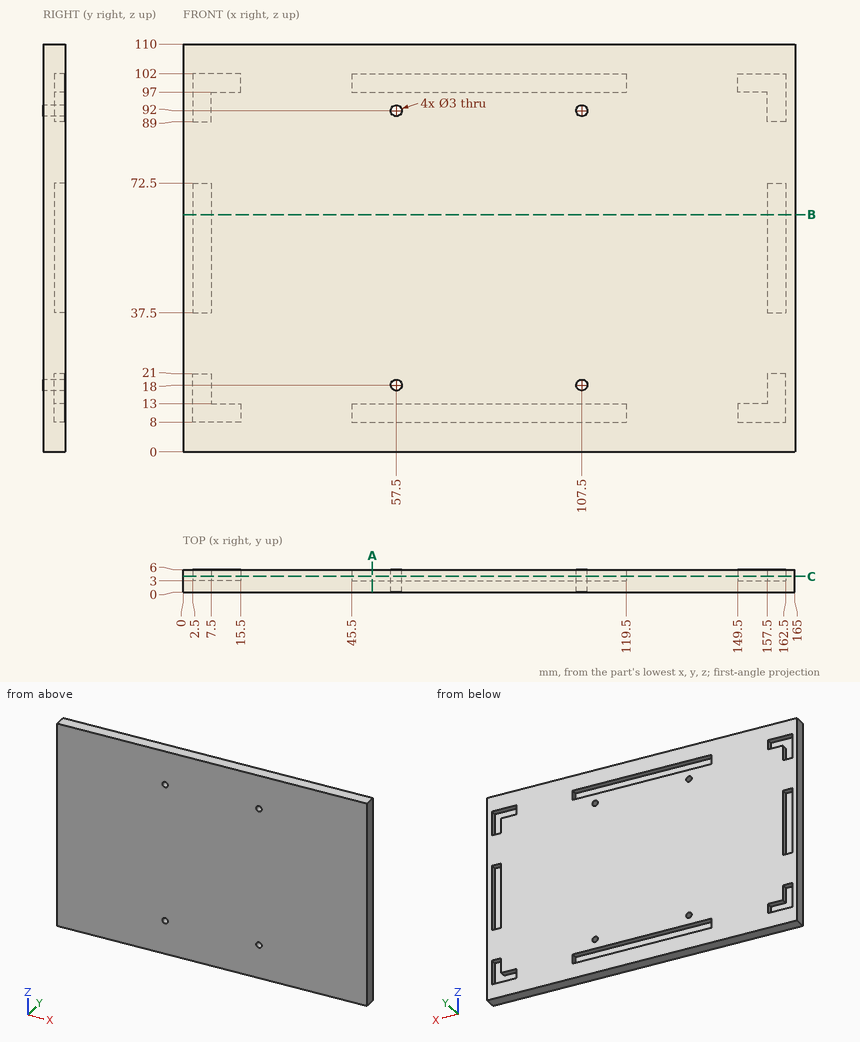
Print and shaded views of the part. All mm, measured from the part's lowest x, y and z. Coordinates: 2 decimals unless noted, no trailing zeros. Loops run counter-clockwise (first coordinate to the right, second up) from the corner with the lowest first, then second, coordinate; pieces in that order, holes last. Notation, with made-up numbers: (40, 75.5) -> (72, 75.5) arc R18 cw to (72, 81.5) -> close; hole circle Ø8 at (50, 37). An arc over 180 degrees is marked (long way). Use one line per item in the form item = value. Start each with the question number.
(1) Flat gauge pin, fed straight in: pin 1 (2.5 mm diameter, centred on x = 76, z = 11, fed in from +Y). Where does the tip first touch, or does it go through?
(2) Probe probe 1 along X at (y, z) = (3.45, 18); probe 2 along X at (y, z) = (2.95, 18); probe 3 along Z at (x, y) = (107.5, 2.4). List the from-to ranges inside material, lowest first. Write a range as from..to.
(3) Cut at B-B on z = 64. Give the cut face in (x, y), and give its area (3 significant figures).
(4) Cut at A-A on x = 51. Give the cut face in (y, z).
(5) Cut at C-C on y = 4.25. Give the number of separate pieces and of enclosed holes in the cut face, and give its area (3 significant figures).
Values:
q1.pin_1 = 3
q2.probe_1 = 0..2.5, 7.5..56, 59..106, 109..157.5, 162.5..165
q2.probe_2 = 0..56, 59..106, 109..165
q2.probe_3 = 0..16.5, 19.5..90.5, 93.5..110
q3.outline = (0, 0) -> (165, 0) -> (165, 6) -> (162.5, 6) -> (162.5, 3) -> (157.5, 3) -> (157.5, 6) -> (7.5, 6) -> (7.5, 3) -> (2.5, 3) -> (2.5, 6) -> (0, 6) -> close
q3.area = 960 mm2
q4.outline = (0, 0) -> (6, 0) -> (6, 8) -> (3, 8) -> (3, 13) -> (6, 13) -> (6, 97) -> (3, 97) -> (3, 102) -> (6, 102) -> (6, 110) -> (0, 110) -> close
q5.separate_pieces = 1
q5.enclosed_holes = 12
q5.area = 16,600 mm2
